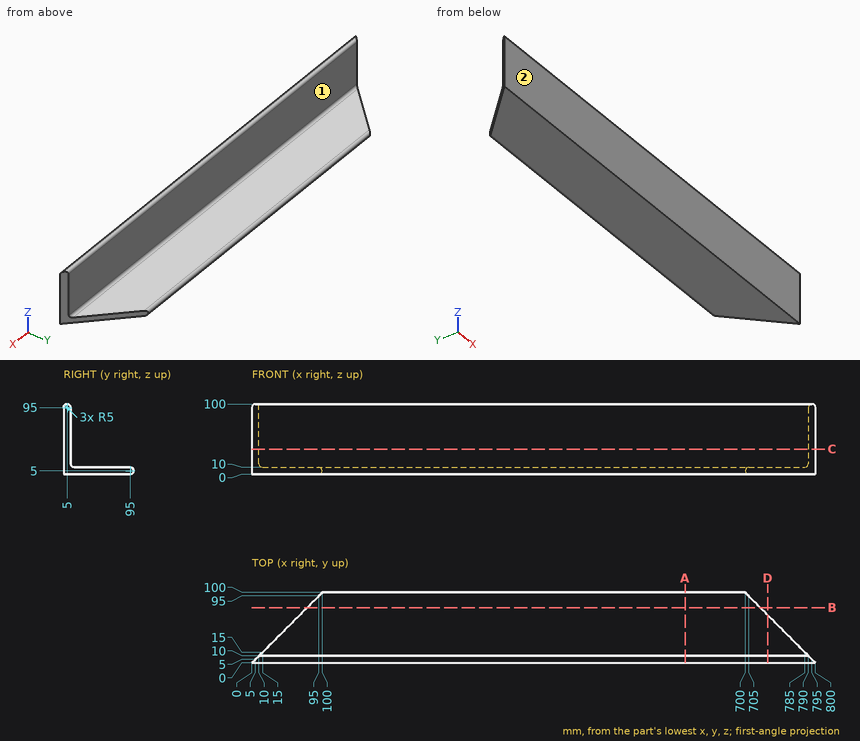
The figure shows three views and two pictorial views of one solid part (mm, origin at its lowest corner). Answer the questions. A direction names the side the tool comes from. Coordinates: 2 decimals unless noted, no trailing zeros. Write each loop counter-clockwise with the first axis right and the second up, starting at its lowest first coordinate (ties: lowest second). Pieces come first, ordered by that corner, then holes. Notation, with made-up numbers: M 33.25,8.25 L 57.25,8.25 A25 ccw 57.25,21.25 Z; hole C 48,50 d4. An arc over 180 degrees is marked long. Answer as CSV lines item,"result". Start each with the question number.
Item 1: Section B-B on y = 78.5 is taken. Write down the section's boundary in (x, z), and give its area (3 significant figures).
Item 2: Section C-C on z = 36 is taken. Write down the section's boundary in (x, y), and give its area (3 significant figures).
Item 3: Section A-A on x = 615 is taken. Write down the section's boundary in (y, z).
Item 4: Consider L1, parallel to Y at x = 374.5, z = 67.5; L2, parallel to Z at x = 349, y = 11.5. Determine where each line is inside the solid, lowest interval first.
Item 5: Section D-D on x = 732 is taken. Write down the section's boundary in (y, z).
Item 6: A tool of negligible diameter and unlimited length cuts with its end or side. For the marked faces 1 and 2, from which of +Z, -Z, +X, -X, +Y, -Y can it reach the whole face along a straight path? Write none if from no direction.
Item 7: Flat-ended cylindrical pins translate along their axes: P1, Ø6, axis at x = 487, y = 29, coming from the +Z side; P2, Ø24, axis at x = 342.5, z = 66.5, coming from the +Y side. Find the tip coordinate at first contact, or state that the pin passes through.
Checks:
1,outline,"M 78.5,0 L 721.5,0 L 721.5,10 L 78.5,10 Z"
1,area,"6,430 mm²"
2,outline,"M 0,0 L 800,0 L 790,10 L 10,10 Z"
2,area,"7,900 mm²"
3,outline,"M 0,0 L 95,0 A5 ccw 95,10 L 15,10 A5 cw 10,15 L 10,95 A5 ccw 0,95 Z"
4,L1,"y = 0 to 10"
4,L2,"z = 0 to 11.43"
5,outline,"M 0,0 L 68,0 L 68,10 L 15,10 A5 cw 10,15 L 10,95 A5 ccw 0,95 Z"
6,face 1,"+Z, +X, -X, +Y"
6,face 2,"+Z, -Z, +X, -X, -Y"
7,P1,"stops at z = 10"
7,P2,"stops at y = 10"
